Here's how the part is built. I have some questions about the finished solid (model axes, mm). A direction names the side the tool comes from. Round coordinates to 2 decimals unless told otherwise and drop trailing zeros. Write each loop counter-clockwise with the first axis right and the second up, starting at its lowest first coordinate (ties: lowest second). Pieces come first, ordered by that corner, then holes. Notation, with made-up numbers: (88, 86) -> (103, 86) arc R22 ccw to (103, 104) -> close; hole circle Ø1 at (-6, 4). An arc over 180 degrees is marked (long way). Answer in a Markdown table with one row per item. Add a question column.
from build123d import *

# Parameters (mm, degrees)
SURFACE_EXTRUDE1_1_BACK  = 4.75
SURFACE_EXTRUDE1_1_DEPTH = 9.5
THICKEN1_T1              = 0.25
FILLET1_R                = 4.75
SKETCH2_W                = 12
SKETCH2_H                = 20
BOSS_EXTRUDE1_DEPTH      = 0.25
FILLET2_R                = 6
FILLET3_R                = 0.5


with BuildPart() as body_1:
    # Surface-Extrude1: a surface, the sketch's curves swept straight by 9.5 mm
    with BuildLine(Plane(origin=(0, 0, 0), x_dir=(0, 0, -1), z_dir=(1, 0, 0)).offset(-SURFACE_EXTRUDE1_1_BACK), mode=Mode.PRIVATE) as surface_extrude1_1_path:
        Line((30.616025404, -5.004809472), (10.616025404, -5.004809472))
        Line((10.616025404, -5.004809472), (6.770725942, -5.004809472))
        ThreePointArc((6.770725942, -5.004809472), (5.770725942, -5.272758664), (5.038675135, -6.004809472))
        Line((5.038675135, -6.004809472), (1.866025404, -11.5))
        ThreePointArc((1.866025404, -11.5), (0.741180955, -11.965925826), (0, -11))
        Line((0, -11), (0, 0))
    surface_extrude1_1 = Shell.extrude(surface_extrude1_1_path.wire(), (1 * SURFACE_EXTRUDE1_1_DEPTH, 0 * SURFACE_EXTRUDE1_1_DEPTH, 0 * SURFACE_EXTRUDE1_1_DEPTH))
    add(Solid.thicken(surface_extrude1_1, THICKEN1_T1))

    # Fillet1
    fillet1_edges = [body_1.edges().sort_by_distance(p)[0] for p in [
        (4.75, 0, 0.125),
        (-4.75, 0, 0.125),
    ]]
    fillet(fillet1_edges, radius=FILLET1_R - 0.0001)  # a hair under: the kernel refuses the full size

    # Sketch2 → Boss-Extrude1 (add)
    with BuildSketch(Plane(origin=(0, -5.004809472, 0), x_dir=(1, 0, 0), z_dir=(0, 1, 0))):
        with Locations((0, 20.616025404)):
            Rectangle(SKETCH2_W, SKETCH2_H)
    extrude(amount=-BOSS_EXTRUDE1_DEPTH)

    # Fillet2
    fillet2_edges = [body_1.edges().sort_by_distance(p)[0] for p in [
        (-6, -5.129809472, -30.616025404),
        (6, -5.129809472, -30.616025404),
    ]]
    fillet(fillet2_edges, radius=FILLET2_R - 0.0001)  # a hair under: the kernel refuses the full size

    # Fillet3
    fillet3_edges = [body_1.edges().sort_by_distance(p)[0] for p in [
        (-6, -5.129809472, -10.616025404),
        (6, -5.129809472, -10.616025404),
    ]]
    fillet(fillet3_edges, radius=FILLET3_R)


solid = body_1.part
Item 1: If we section it at D-D on y = -3.75: Please give me the cut outline in (x, z), then the cut area to 3 significant figures.
Item 2: I need wall thicknesses on line 1 along Z through (x, y) = (-0.5, -6.5); line 2 along Y through (x, z) = (0.25, -17.5); line 3 along Z through (x, y) = (-2.5, -1.25). Which ranges of each line are inside material? Lowest first, please. Write a range as from..to.
Item 3: If we section it at C-C on z = -20: Please give me the cut outline in (x, y), then the cut area to 3 significant figures.
Item 4: If we section it at A-A on x = -1.25: Please give me the cut outline in (y, z) (3 decimals), then the cut area to 3 significant figures.
Item 5: On a 3-axis mill with a long thin cutter (end or side, diameter ignored), from which of +Z, -Z, +X, -X, +Y, -Y can I reach the whole of each face in a straight line? I mean faces 1 (the flat face through (-0.067, -8.714, -3.475)), 2 (the cylindrical face through (-0.067, -12.213, -0.699)), 3 (the flat face through (0, -5.255, -19)). Say none if no direction works.
Item 6: If we mould it in two halves opening along Z, with no side actions, what happens to faces 4 (the cylindrical face through (-0.07, -5.48, -5.91)), 5 (the flat face through (0, -5.005, -19)), 6 (the cylindrical face through (-0.067, -5.265, -5.783))? For each: pulls with the +Z half, pulls with the -Z half, needs draft (parallel to the pull), parting line crosses it, or undercut.
Item 7: If we section it at B-B on y = -10.5: Please give me the cut outline in (x, z), then the cut area to 3 significant figures.
Item 8: For P1, Ø1.5, axis at x = -3.5, z = -13, coming from the +Y side; P2, Ø4, axis at y = -6.5, z = -6, coming from the -X side; P3, Ø6, axis at x = -0.5, z = -21, coming from the -Y side, each with a flat end and sliding along its axis, tell me the tip position at first contact or that it passes through.
Results list:
| question | item | result |
|---|---|---|
| 1 | outline | (-4.64, 0) -> (4.64, 0) -> (4.64, 0.25) -> (-4.64, 0.25) -> close |
| 1 | area | 2.32 mm² |
| 2 | line 1 | -5.04..-4.75, 0..0.25 |
| 2 | line 2 | -5.25..-5 |
| 2 | line 3 | 0..0.25 |
| 3 | outline | (-6, -5.25) -> (6, -5.25) -> (6, -5) -> (-6, -5) -> close |
| 3 | area | 3.00 mm² |
| 4 | outline | (-11.625, -2.083) -> (-6.13, -5.255) arc R1.75 cw to (-5.255, -6.771) -> (-5.255, -30.484) -> (-5.005, -30.484) -> (-5.005, -6.771) arc R2 ccw to (-6.005, -5.039) -> (-11.5, -1.866) arc R1 cw to (-11, 0) -> (-0.167, 0) -> (-0.167, 0.25) -> (-11, 0.25) arc R1.25 ccw to start |
| 4 | area | 11.5 mm² |
| 5 | face 1 | +X, -X, +Y |
| 5 | face 2 | +X, -X, -Y |
| 5 | face 3 | -Z, +X, -X, -Y |
| 6 | face 4 | pulls with the -Z half |
| 6 | face 5 | needs draft |
| 6 | face 6 | undercut |
| 7 | outline | (-4.75, -2.73) -> (4.75, -2.73) -> (4.75, -2.44) -> (-4.75, -2.44) -> close; (-4.75, 0) -> (4.75, 0) -> (4.75, 0.25) -> (-4.75, 0.25) -> close |
| 7 | area | 5.12 mm² |
| 8 | P1 | y = -5 |
| 8 | P2 | x = -4.75 |
| 8 | P3 | y = -5.25 |
